from build123d import *

# Parameters (mm, degrees)
SKETCH_R        = 30
PAD_DEPTH       = 40
POCKET_DEPTH    = 35
SKETCH002_R     = 19.5
POCKET001_DEPTH = 35
CHAMFER_SIZE    = 4
CHAMFER001_SIZE = 2


with BuildPart() as part:
    # Sketch → Pad (new body)
    with BuildSketch(Plane.XY):
        Circle(SKETCH_R)
    extrude(amount=PAD_DEPTH)

    # Sketch001 (on Face3 of Pad) → Pocket (cut)
    with BuildSketch(Plane.XY.offset(40)):
        Polygon((-16.5, 16.5), (16.5, 16.5), (16.5, -16.5), (13.5, -16.5), (13.5, 13.5), (-16.5, 13.5), align=None)
    extrude(amount=-POCKET_DEPTH, mode=Mode.SUBTRACT)

    # Sketch002 (on Face3 of Pocket) → Pocket001 (cut)
    with BuildSketch(Plane.XY.offset(40)):
        Circle(SKETCH002_R)
    extrude(amount=-POCKET001_DEPTH, mode=Mode.SUBTRACT)

    # Chamfer
    chamfer_edges = [part.edges().sort_by_distance(p)[0] for p in [
        (-30, 0, 40),
    ]]
    chamfer(chamfer_edges, length=CHAMFER_SIZE)

    # Chamfer001
    chamfer001_edges = [part.edges().sort_by_distance(p)[0] for p in [
        (-30, 0, 0),
    ]]
    chamfer(chamfer001_edges, length=CHAMFER001_SIZE)


solid = part.part
Verification items for the finished model (mm, model axes). A direction names the side the tool comes from. Coordinates: 2 decimals unless noted, no trailing zeros. Loops run counter-clockwise (first coordinate to the right, second up) from the corner with the lowest first, then second, coordinate; pieces in that order, holes last. Notation, with made-up numbers: M -3,55 L 12,55 A26 cw 12,69 Z; hole C 31.5,-20.5 d2. An arc over 180 degrees is marked long. One line per item, written item: value.
1. Set-up check for faces 1 (the flat face through (17, -10, 40)), 2 (the flat face through (13, 16.5, 23)): record each of +Z, -Z, +X, -X, +Y, -Y from which the full face is reachable in a straight line by a thin tool's end or side.
Answers follow:
face 1: +Z, +X, -X, +Y, -Y
face 2: +Z
2. Mould release check, pull along X, two halves, no side actions. Record for faces 3 (the flat face through (-15, 13.5, 23)), 4 (the conical face through (12.087, -23.239, 39.806)), 5 (the flat face through (0, 0, 0)): pulls with the +X half, pulls with the -X half, needs draft (parallel to the pull), parting line crosses it, or undercut.
Answers follow:
face 3: undercut
face 4: parting line crosses it
face 5: needs draft
3. Gauge pin test, flat ends, axial feed: P1, Ø5, axis at x = -9, z = 15.5, coming from the +Y side; P2, Ø1.2, axis at y = -15.5, z = 28, coming from the +X side; P3, Ø5, axis at x = -23.5, z = 13, coming from the +Y side. Record the tip position at first contact, or that the pin passes through.
Answers follow:
P1: y = 29.29
P2: x = 26.04
P3: y = 21.42
4. Section check A-A on z = 31.5. Record the cut outline in (x, y), plus the area to 3 significant figures.
Answers follow:
outline: C 0,0 d60; hole M -16.5,13.5 L -14.07,13.5 A19.5 ccw 13.5,-14.07 L 13.5,-16.5 L 16.5,-16.5 L 16.5,-10.39 A19.5 ccw 16.5,10.39 L 16.5,16.5 L 10.39,16.5 A19.5 ccw -10.39,16.5 L -16.5,16.5 Z
area: 1,590 mm^2
5. Material ranges on line 1 along Y through (x, z) = (-16, 38); line 2 along Y through (x, z) = (11.5, 17); line 3 along Y through (x, z) = (8, 38.5), recorded low to high. Write a range as from..to.
Answers follow:
line 1: -22.98..-11.15, 11.15..13.5, 16.5..22.98
line 2: -27.71..-15.75, 16.5..27.71
line 3: -26.31..-17.78, 17.78..26.31
6. Section check B-B on x = 0. Record the cut outline in (y, z).
Answers follow:
outline: M -30,2 L -28,0 L 28,0 L 30,2 L 30,36 L 26,40 L 19.5,40 L 19.5,5 L -19.5,5 L -19.5,40 L -26,40 L -30,36 Z
